For this review, take the finished solid that the model builds, in its own axes (mm). Coordinates: 2 decimals unless noted, no trailing zeros. Write each loop counter-clockwise with the first axis right and the second up, starting at its lowest first coordinate (ties: lowest second). Pieces come first, ordered by that corner, then holes. Notation, with made-up numbers: M 17.5,65.5 L 25.5,65.5 A22 ccw 25.5,89.5 Z; hole C -5.75,21 d6. An arc over 180 degrees is marked long. Return JSON: item names as keys, results as strings.
```python
from build123d import *

# Parameters (mm, degrees)
SKETCH1_W                                         = 42
SKETCH1_H                                         = 65
BOSS_EXTRUDE1_DEPTH                               = 15.875
SKETCH2_R                                         = 1
CUT_EXTRUDE1_DEPTH                                = 1
CUT_EXTRUDE1_DEPTH_BACK                           = 1
CSK_FOR_8_FLAT_HEAD_MACHINE_SCREW_100_D           = 4.4958
CSK_FOR_8_FLAT_HEAD_MACHINE_SCREW_100_CSINK_D     = 8.4328
CSK_FOR_8_FLAT_HEAD_MACHINE_SCREW_100_CSINK_ANGLE = 100


with BuildPart() as part:
    # Sketch1 → Boss-Extrude1 (new body)
    with BuildSketch(Plane.XY):
        Rectangle(SKETCH1_W, SKETCH1_H)
    extrude(amount=BOSS_EXTRUDE1_DEPTH)

    # Sketch2 → Cut-Extrude1 (cut, two sides)
    with BuildSketch(Plane.XY.offset(15.875)) as cut_extrude1_sk:
        with Locations((-13.459539776, -6.5)):
            Circle(SKETCH2_R)
        with Locations((-13.459539776, 17)):
            Circle(SKETCH2_R)
        with Locations((13.459539776, 17)):
            Circle(SKETCH2_R)
        with Locations((13.459539776, -6.5)):
            Circle(SKETCH2_R)
    extrude(amount=CUT_EXTRUDE1_DEPTH, mode=Mode.SUBTRACT)
    extrude(cut_extrude1_sk.sketch, amount=-CUT_EXTRUDE1_DEPTH_BACK, mode=Mode.SUBTRACT)

    # CSK for #8 Flat Head Machine Screw (100)1 (through all)
    with Locations(Plane.XY.offset(15.875)):
        with Locations((0, 15.875), (0, -15.875)):
            CounterSinkHole(CSK_FOR_8_FLAT_HEAD_MACHINE_SCREW_100_D / 2, CSK_FOR_8_FLAT_HEAD_MACHINE_SCREW_100_CSINK_D / 2, counter_sink_angle=CSK_FOR_8_FLAT_HEAD_MACHINE_SCREW_100_CSINK_ANGLE)


solid = part.part
```
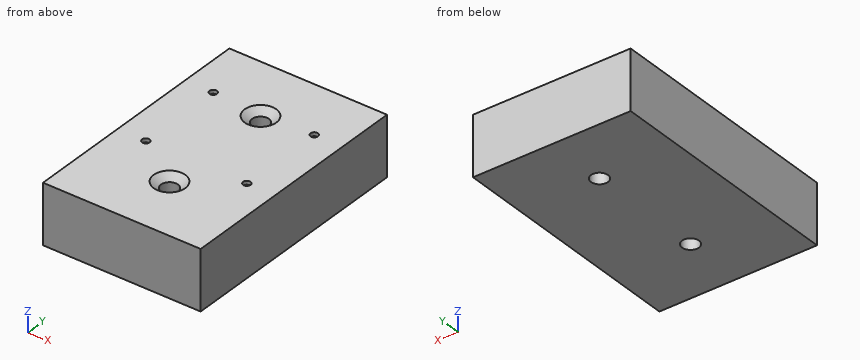
1. Wall thickness on L1, parallel to Y at x = 0, z = 8; L2, parallel to Y at x = -0.5, z = 10; L3, parallel to X at y = 14, z = 8: over which ranges is each line inside the solid? List them lowest first. Write a range as from..to.
Checks:
{"L1": "-32.5..-18.12, -13.63..13.63, 18.12..32.5", "L2": "-32.5..-18.07, -13.68..13.68, 18.07..32.5", "L3": "-21..-1.24, 1.24..21"}
2. We need section A-A (x = 0). State the section outline as (y, z) points (3 decimals), plus the area to 3 significant figures.
Checks:
{"outline": "M -32.5,0 L -18.123,0 L -18.123,14.223 L -20.091,15.875 L -32.5,15.875 Z; M -13.627,0 L 13.627,0 L 13.627,14.223 L 11.659,15.875 L -11.659,15.875 L -13.627,14.223 Z; M 18.123,0 L 32.5,0 L 32.5,15.875 L 20.091,15.875 L 18.123,14.223 Z", "area": "883 mm2"}
3. Clearance check with flat-ended pins moving along their axes: pin 1 Ø5 at (x, y) = (0, -15.875) entering from +Z; pin 2 Ø0.6 at (x, y) = (-13.5, 17) entering from +Z (3 decimals). State where each tip first meets the part, or that it passes through.
Checks:
{"pin 1": "z = 14.43", "pin 2": "z = 14.875"}
